Verification items for the finished model (mm, model axes). Face numbers are marked on the shaded views. A direction names the side the tool comes from. Round coordinates to 2 decimals unless told otherwise and drop trailing zeros. Write each loop counter-clockwise with the first axis right and the second up, starting at its lowest first coordinate (ties: lowest second). Pieces come first, ordered by that corner, then holes. Notation, with made-up numbers: (47, 72) -> (85, 72) arc R12 cw to (85, 85) -> close; hole circle Ø4 at (35, -28). An arc over 180 degrees is marked (long way). Use CSV: the item, a comma, the result in double quotes.
```python
from build123d import *

# Parameters (mm, degrees)
EXTRUDE_RATCHET_EDGE_DEPTH      = 10
PATTERN_EDGE_TO_FORM_GEAR_COUNT = 26
GEAR_FACE_DEPTH                 = 5
PCB_INSET_DEPTH                 = 1
SKETCH7_R                       = 6.35
CUT_BEARING_HOLE_DEPTH          = 5
PCB_INSET_REAR_DEPTH            = 1
PIN_HOLES_R                     = 0.6
PIN_HOLES_CUT_DEPTH             = 15
SKETCH15_R                      = 5.18
CUT_EXTRUDE3_DEPTH              = 16


with BuildPart() as part:
    # Sketch1 → Extrude ratchet edge (new body)
    with BuildSketch(Plane(origin=(0, 0, 0), x_dir=(1, 0, 0), z_dir=(0, 1, 0))):
        with BuildLine():
            Line((0, 0), (29.613725431, 7.299127761))
            ThreePointArc((29.613725431, 7.299127761), (31.486736206, 3.871832194), (32, 0))
            Line((32, 0), (0, 0))
        make_face()
    extrude_ratchet_edge = extrude(amount=EXTRUDE_RATCHET_EDGE_DEPTH)

    # Pattern edge to form gear: Extrude ratchet edge ×26 about axis
    pattern_edge_to_form_gear_axis = Axis((0, 0, 0), (0, 1, 0))
    for i in range(1, PATTERN_EDGE_TO_FORM_GEAR_COUNT):
        add(extrude_ratchet_edge.rotate(pattern_edge_to_form_gear_axis, i * 360 / PATTERN_EDGE_TO_FORM_GEAR_COUNT))

    # Sketch12 → Gear face (add)
    with BuildSketch(Plane(origin=(0, 10, 0), x_dir=(1, 0, 0), z_dir=(0, 1, 0))):
        with BuildLine():
            Line((28.927375325, -2.125741727), (29.026395325, -2.515151727))
            Line((29.026395325, -2.515151727), (29.142735325, -2.671831727))
            Line((29.142735325, -2.671831727), (29.262305325, -2.787261727))
            Line((29.262305325, -2.787261727), (29.383725325, -2.880131727))
            Line((29.383725325, -2.880131727), (29.624225325, -3.082071727))
            Line((29.624225325, -3.082071727), (29.879175325, -3.139941727))
            Line((29.879175325, -3.139941727), (30.384275325, -3.299211727))
            Line((30.384275325, -3.299211727), (30.884385325, -3.499611727))
            Line((30.884385325, -3.499611727), (31.379885325, -3.733371727))
            Line((31.379885325, -3.733371727), (31.870755325, -3.996551727))
            Line((31.870755325, -3.996551727), (32.356805325, -4.286661727))
            Line((32.356805325, -4.286661727), (32.837785325, -4.602001727))
            Line((32.837785325, -4.602001727), (33.313375325, -4.941291727))
            Line((33.313375325, -4.941291727), (33.783255325, -5.303521727))
            Line((33.783255325, -5.303521727), (33.502035325, -6.859281727))
            Line((33.502035325, -6.859281727), (32.935085325, -7.034091727))
            Line((32.935085325, -7.034091727), (32.370805325, -7.185411727))
            Line((32.370805325, -7.185411727), (31.809875325, -7.312411727))
            Line((31.809875325, -7.312411727), (31.253015325, -7.414011727))
            Line((31.253015325, -7.414011727), (30.701075325, -7.488691727))
            Line((30.701075325, -7.488691727), (30.155095325, -7.534201727))
            Line((30.155095325, -7.534201727), (29.616475325, -7.546831727))
            Line((29.616475325, -7.546831727), (29.087575325, -7.519191727))
            Line((29.087575325, -7.519191727), (28.828505325, -7.484151727))
            Line((28.828505325, -7.484151727), (28.532525325, -7.589111727))
            Line((28.532525325, -7.589111727), (28.386275325, -7.633601727))
            Line((28.386275325, -7.633601727), (28.233865325, -7.699871727))
            Line((28.233865325, -7.699871727), (28.070045325, -7.805911727))
            Line((28.070045325, -7.805911727), (27.840955325, -8.136001727))
            Line((27.840955325, -8.136001727), (27.578045325, -8.986971727))
            ThreePointArc((27.578045325, -8.986971727), (-28.554449146, 5.09486788), (28.984351964, -1.105253821))
            Line((28.984351964, -1.105253821), (28.927375325, -2.125741727))
        make_face()
    extrude(amount=GEAR_FACE_DEPTH)

    # Sketch10 → PCB inset (cut)
    with BuildSketch(Plane(origin=(0, 15, 0), x_dir=(1, 0, 0), z_dir=(0, 1, 0))):
        with BuildLine():
            Line((-0.753755436, 29.351723584), (-0.753755436, 27.351723584))
            ThreePointArc((-0.753755436, 27.351723584), (0.246244564, -27.630088583), (1.246244564, 27.351723584))
            Line((1.246244564, 27.351723584), (1.246244564, 29.351723584))
            Line((1.246244564, 29.351723584), (-0.753755436, 29.351723584))
        make_face()
    extrude(amount=-PCB_INSET_DEPTH, mode=Mode.SUBTRACT)

    # Sketch7 → Cut bearing hole (cut)
    with BuildSketch(Plane(origin=(0, 15, 0), x_dir=(1, 0, 0), z_dir=(0, 1, 0))):
        Circle(SKETCH7_R)
    extrude(amount=-CUT_BEARING_HOLE_DEPTH, mode=Mode.SUBTRACT)

    # Sketch11 → PCB inset rear (cut)
    with BuildSketch(Plane.XZ):
        with BuildLine():
            Line((1, -29.481812167), (1, -27.481812167))
            ThreePointArc((1, -27.481812167), (0, 27.5), (-1, -27.481812167))
            Line((-1, -27.481812167), (-1, -29.481812167))
            Line((-1, -29.481812167), (1, -29.481812167))
        make_face()
    extrude(amount=-PCB_INSET_REAR_DEPTH, mode=Mode.SUBTRACT)

    # pin holes → Pin holes cut (cut, through all)
    with BuildSketch(Plane(origin=(0, 14, 0), x_dir=(1, 0, 0), z_dir=(0, 1, 0))):
        with Locations((15, 0)):
            Circle(PIN_HOLES_R)
        with Locations((14.564127261, -3.589734964)):
            Circle(PIN_HOLES_R)
        with Locations((13.281840385, -6.970847581)):
            Circle(PIN_HOLES_R)
        with Locations((11.227661223, -9.946839874)):
            Circle(PIN_HOLES_R)
        with Locations((8.520971201, -12.344757988)):
            Circle(PIN_HOLES_R)
        with Locations((5.319073306, -14.02524364)):
            Circle(PIN_HOLES_R)
        with Locations((1.808050204, -14.890633111)):
            Circle(PIN_HOLES_R)
        with Locations((-1.808050204, -14.890633111)):
            Circle(PIN_HOLES_R)
        with Locations((-5.319073306, -14.02524364)):
            Circle(PIN_HOLES_R)
        with Locations((-8.520971201, -12.344757988)):
            Circle(PIN_HOLES_R)
        with Locations((-11.227661223, -9.946839874)):
            Circle(PIN_HOLES_R)
        with Locations((-13.281840385, -6.970847581)):
            Circle(PIN_HOLES_R)
        with Locations((-14.564127261, -3.589734964)):
            Circle(PIN_HOLES_R)
        with Locations((-15, 0)):
            Circle(PIN_HOLES_R)
        with Locations((-14.564127261, 3.589734964)):
            Circle(PIN_HOLES_R)
        with Locations((-13.281840385, 6.970847581)):
            Circle(PIN_HOLES_R)
        with Locations((-11.227661223, 9.946839874)):
            Circle(PIN_HOLES_R)
        with Locations((-8.520971201, 12.344757988)):
            Circle(PIN_HOLES_R)
        with Locations((-5.319073306, 14.02524364)):
            Circle(PIN_HOLES_R)
        with Locations((-1.808050204, 14.890633111)):
            Circle(PIN_HOLES_R)
        with Locations((1.808050204, 14.890633111)):
            Circle(PIN_HOLES_R)
        with Locations((5.319073306, 14.02524364)):
            Circle(PIN_HOLES_R)
        with Locations((8.520971201, 12.344757988)):
            Circle(PIN_HOLES_R)
        with Locations((11.227661223, 9.946839874)):
            Circle(PIN_HOLES_R)
        with Locations((13.281840385, 6.970847581)):
            Circle(PIN_HOLES_R)
        with Locations((14.564127261, 3.589734964)):
            Circle(PIN_HOLES_R)
    extrude(amount=-PIN_HOLES_CUT_DEPTH, mode=Mode.SUBTRACT)

    # Sketch15 → Cut-Extrude3 (cut, through all)
    with BuildSketch(Plane.XZ):
        Circle(SKETCH15_R)
    extrude(amount=-CUT_EXTRUDE3_DEPTH, mode=Mode.SUBTRACT)


solid = part.part
```
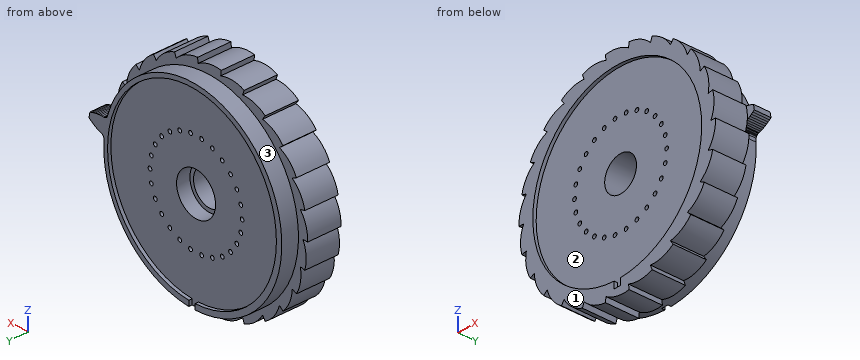
Q1. Material ranges on L1, parallel to Z at x = 8, y = 1.25; L2, parallel to Z at x = 8, y = 10.25; L3, parallel to Y at x = -27.5, z = -12.5, recorded low to high.
Filled in:
L1,"-30.78 to -12.64, -12.05 to 12.05, 12.64 to 30.61"
L2,"-27.88 to -12.64, -12.05 to 12.05, 12.64 to 27.88"
L3,"0 to 10"
Q2. Access from +Z, -Z, +X, -X, +Y, -Y to the whole of each face (thin tool, end or side, straight path). Record for the marked faces 1, 2 and 3.
Filled in:
face 1,"+Z, -Z, +X, -X, -Y"
face 2,"-Y"
face 3,"+Y"
Q3. Section check B-B (y = 6.5). State how many separate pieces and enclosed holes the cut face has, plus the area to 3 significant figures.
Filled in:
separate pieces,"1"
enclosed holes,"27"
area,"3,020 mm²"
Q4. Section check C-C (x = -16.5). Record the cut outline in (y, z), plus the area to 3 significant figures.
Filled in:
outline,"(0, -26.33) -> (10, -26.33) -> (10, -23.86) -> (15, -23.86) -> (15, -21.68) -> (14, -21.68) -> (14, 21.94) -> (15, 21.94) -> (15, 23.86) -> (10, 23.86) -> (10, 27.4) -> (0, 27.4) -> (0, 22) -> (1, 22) -> (1, -22) -> (0, -22) -> close"
area,"688 mm²"
Q5. Section check A-A (x = 0). Record the cut outline in (y, z), plus the area to 3 significant figures.
Filled in:
outline,"(0, -31.73) -> (10, -31.73) -> (10, -29.01) -> (14, -29.01) -> (14, -6.35) -> (10, -6.35) -> (10, -5.18) -> (1, -5.18) -> (1, -29.48) -> (0, -29.48) -> close; (0, 27.5) -> (1, 27.5) -> (1, 5.18) -> (10, 5.18) -> (10, 6.35) -> (14, 6.35) -> (14, 27.63) -> (15, 27.63) -> (15, 29.01) -> (10, 29.01) -> (10, 31.73) -> (0, 31.73) -> close"
area,"667 mm²"
Q6. Go/stop test with flat-tipped pins: P1, Ø8, axis at y = 8, z = -25, coming from the -X side; P2, Ø1, axis at y = 7.5, z = -19, coming from the +X side; P3, Ø1.6, axis at x = -14.56, z = -3.59, coming from the -Y side. Record where each tip stops, or that it passes through.
Filled in:
P1,"x = -24.16"
P2,"x = 25.6"
P3,"y = 1"
